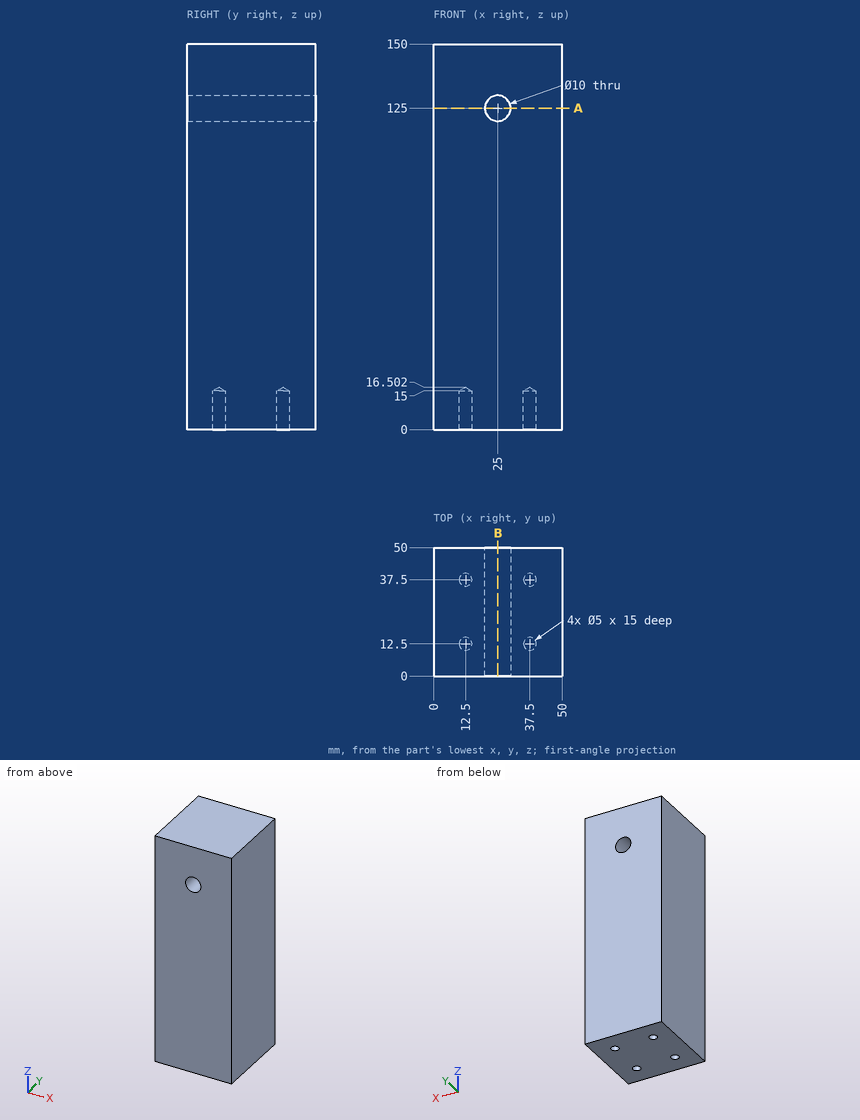
Can you work these out from the drawing? Everything is in mm from the part's minimum corner. Round coordinates to 2 decimals unless told otherwise and drop trailing zeros. Order: outer loops, then holes, each group sorted by start corner. A loop starts at its lowest first (then second) coordinate and runs counter-clockwise, first axis right, second up. Notation, with made-up numbers: (22, 66) - (67, 66) arc R23 ccw to (67, 81) - close; hole circle Ø3 at (-19.5, -26). An arc over 180 degrees is marked (long way). Answer in a Markdown table with one row per item.
(1) Suppose I cut it at B-B, the plane x = 25. Please give me the cut outline in (y, z).
From the geometry:
| item | result |
|---|---|
| outline | (0, 0) - (50, 0) - (50, 120) - (0, 120) - close; (0, 130) - (50, 130) - (50, 150) - (0, 150) - close |
(2) For P1, Ø1.5, axis at x = 14, y = 18.5, coming from the -Z side; P2, Ø3, axis at x = 37.5, y = 12.5, coming from the -Z side, each with a flat end and sliding along its axis, tell me the tip position at first contact or that it passes through.
From the geometry:
| item | result |
|---|---|
| P1 | stops at z = 0 |
| P2 | stops at z = 15.6 |
(3) Please list where these lines run through material, in increasing order: L1, parallel to Y at x = 37.5, z = 9.25; L2, parallel to Z at x = 25, y = 23.5. Write a range as from..to.
From the geometry:
| item | result |
|---|---|
| L1 | y = 0..10, 15..35, 40..50 |
| L2 | z = 0..120, 130..150 |
(4) Suppose I cut it at A-A, the plane z = 125. Please give me the cut outline in (x, y), plus the area to 3 significant figures.
From the geometry:
| item | result |
|---|---|
| outline | (0, 0) - (20, 0) - (20, 50) - (0, 50) - close; (30, 0) - (50, 0) - (50, 50) - (30, 50) - close |
| area | 2,000 mm2 |
